```python
from build123d import *

# Parameters (mm, degrees)
SKETCH_1_W          = 10
SKETCH_1_H          = 5
SKETCH_1_W_2        = 30
EXTRUDE_1_DEPTH     = 5
SKETCH_1_3_W        = 10
SKETCH_1_3_H        = 5
SKETCH_1_3_W_2      = 30
EXTRUDE_2_DEPTH     = 85
SKETCH_2_R          = 3
CUT_EXTRUDE_1_DEPTH = 144
FILLET_1_R          = 40
SKETCH_4_W          = 30
SKETCH_4_H          = 5.8
CUT_EXTRUDE_2_DEPTH = 144
SKETCH_5_W          = 60
SKETCH_5_H          = 60
CUT_EXTRUDE_3_DEPTH = 144
SKETCH_6_R          = 5
CUT_EXTRUDE_4_DEPTH = 144


with BuildPart() as part:
    # Sketch 1 → Extrude 1 (new body)
    with BuildSketch(Plane.XY):
        Polygon((0, 42.6), (0, 0), (95, 0), (95, 47.6), (10, 47.6), (10, 42.6), align=None)
        Polygon((10, -42.6), (10, -47.6), (35, -47.6), (75, -47.6), (90, -47.6), (95, -47.6), (95, 0), (0, 0), (0, -42.6), align=None)
        Polygon((35, -47.6), (10, -47.6), (0, -47.6), (0, -52.6), (10, -52.6), (90, -52.6), (95, -52.6), (95, -47.6), (90, -47.6), (75, -47.6), align=None)
        with Locations((5, -45.1)):
            Rectangle(SKETCH_1_W, SKETCH_1_H)
        with Locations((-15, -45.1)):
            Rectangle(SKETCH_1_W_2, SKETCH_1_H)
        Polygon((10, -52.6), (0, -52.6), (-30, -52.6), (-30, -57.6), (10, -57.6), align=None)
        with Locations((-15, 45.1)):
            Rectangle(SKETCH_1_W_2, SKETCH_1_H)
        Polygon((-30, 52.6), (0, 52.6), (10, 52.6), (10, 57.6), (-30, 57.6), align=None)
        Polygon((0, 52.6), (0, 47.6), (10, 47.6), (95, 47.6), (95, 52.6), (10, 52.6), align=None)
        with Locations((5, 45.1)):
            Rectangle(SKETCH_1_W, SKETCH_1_H)
    extrude(amount=-EXTRUDE_1_DEPTH)

    # Sketch 1_3 → Extrude 2 (add)
    with BuildSketch(Plane.XY):
        Polygon((0, 52.6), (0, 47.6), (10, 47.6), (95, 47.6), (95, 52.6), (10, 52.6), align=None)
        Polygon((-30, 52.6), (0, 52.6), (10, 52.6), (10, 57.6), (-30, 57.6), align=None)
        with Locations((5, 45.1)):
            Rectangle(SKETCH_1_3_W, SKETCH_1_3_H)
        with Locations((-15, 45.1)):
            Rectangle(SKETCH_1_3_W_2, SKETCH_1_3_H)
        with Locations((5, -45.1)):
            Rectangle(SKETCH_1_3_W, SKETCH_1_3_H)
        with Locations((-15, -45.1)):
            Rectangle(SKETCH_1_3_W_2, SKETCH_1_3_H)
        Polygon((10, -52.6), (0, -52.6), (-30, -52.6), (-30, -57.6), (10, -57.6), align=None)
        Polygon((35, -47.6), (10, -47.6), (0, -47.6), (0, -52.6), (10, -52.6), (90, -52.6), (95, -52.6), (95, -47.6), (90, -47.6), (75, -47.6), align=None)
    extrude(amount=EXTRUDE_2_DEPTH)

    # Sketch 2 → Cut-Extrude 1 (cut)
    with BuildSketch(Plane.XZ.offset(52.6)):
        with Locations(Location((55, 60, 0), (0, 0, 270))):
            Circle(SKETCH_2_R)
    extrude(amount=-CUT_EXTRUDE_1_DEPTH, mode=Mode.SUBTRACT)

    # Fillet 1
    fillet_1_edges = [part.edges().sort_by_distance(p)[0] for p in [
        (95, -50.1, 85),
        (95, 50.1, 85),
    ]]
    fillet(fillet_1_edges, radius=FILLET_1_R)

    # Sketch 4 → Cut-Extrude 2 (cut)
    with BuildSketch(Plane.XY.offset(85)):
        with Locations((-15, -50.1)):
            Rectangle(SKETCH_4_W, SKETCH_4_H)
        with Locations((-15, 50.1)):
            Rectangle(SKETCH_4_W, SKETCH_4_H)
    extrude(amount=-CUT_EXTRUDE_2_DEPTH, mode=Mode.SUBTRACT)

    # Sketch 5 → Cut-Extrude 3 (cut)
    with BuildSketch(Plane.XY):
        with Locations((45, 0)):
            Rectangle(SKETCH_5_W, SKETCH_5_H)
    extrude(amount=-CUT_EXTRUDE_3_DEPTH, mode=Mode.SUBTRACT)

    # Sketch 6 → Cut-Extrude 4 (cut)
    with BuildSketch(Plane.XZ.offset(57.6)):
        with Locations(Location((-10, 40, 0), (0, 0, 270))):
            Circle(SKETCH_6_R)
        with Locations(Location((-10, 65, 0), (0, 0, 270))):
            Circle(SKETCH_6_R)
        with Locations(Location((-10, 15, 0), (0, 0, 270))):
            Circle(SKETCH_6_R)
    extrude(amount=-CUT_EXTRUDE_4_DEPTH, mode=Mode.SUBTRACT)


solid = part.part
```
Design review of the part built by this model. Coordinates are the model's own, in mm. A direction names the side the tool comes from. Round coordinates to 2 decimals unless told otherwise and drop trailing zeros. Write each loop counter-clockwise with the first axis right and the second up, starting at its lowest first coordinate (ties: lowest second). Pieces come first, ordered by that corner, then holes. Notation, with made-up numbers: (32, -39) -> (76, -39) arc R30 ccw to (76, -17) -> close; hole circle Ø2 at (-3.5, 6). An arc over 180 degrees is marked (long way). Answer in a Markdown table with one row per item.
Q1. Take a section at C-C, the plane x = -19.5. State the section outline as (y, z) points, then the cut area to 3 significant figures.
The answers:
| item | result |
|---|---|
| outline | (-57.6, -5) -> (-53, -5) -> (-53, 85) -> (-57.6, 85) -> close; (-47.2, -5) -> (-42.6, -5) -> (-42.6, 85) -> (-47.2, 85) -> close; (42.6, -5) -> (47.2, -5) -> (47.2, 85) -> (42.6, 85) -> close; (53, -5) -> (57.6, -5) -> (57.6, 85) -> (53, 85) -> close |
| area | 1,660 mm² |
Q2. Clearance check with flat-ended pins moving along their axes: pin 1 Ø5.5 at (y, z) = (-3.5, -1.5) entering from -X; pin 2 Ø4 at (x, z) = (49, -3) entering from +Y; pin 3 Ø3 at (x, z) = (68, 16.5) entering from -Y. State where each tip first meets the part, or that it passes through.
The answers:
| item | result |
|---|---|
| pin 1 | x = 0 |
| pin 2 | y = 52.6 |
| pin 3 | y = -52.6 |
Q3. Take a section at A-A, the plane x = 26. State the section outline as (y, z) points, then the cut area to 3 significant figures.
The answers:
| item | result |
|---|---|
| outline | (-52.6, -5) -> (-30, -5) -> (-30, 0) -> (-47.6, 0) -> (-47.6, 85) -> (-52.6, 85) -> close; (30, -5) -> (52.6, -5) -> (52.6, 85) -> (47.6, 85) -> (47.6, 0) -> (30, 0) -> close |
| area | 1,080 mm² |
Q4. Take a section at D-D, the plane z = 78. State the section outline as (x, y) points.
The answers:
| item | result |
|---|---|
| outline | (-30, -57.6) -> (10, -57.6) -> (10, -52.6) -> (77.61, -52.6) -> (77.61, -47.6) -> (10, -47.6) -> (10, -42.6) -> (-30, -42.6) -> (-30, -47.2) -> (0, -47.2) -> (0, -53) -> (-30, -53) -> close; (-30, 42.6) -> (10, 42.6) -> (10, 47.6) -> (77.61, 47.6) -> (77.61, 52.6) -> (10, 52.6) -> (10, 57.6) -> (-30, 57.6) -> (-30, 53) -> (0, 53) -> (0, 47.2) -> (-30, 47.2) -> close |
Q5. Take a section at B-B, the plane y = 16. State the section outline as (x, z) points.
The answers:
| item | result |
|---|---|
| outline | (0, -5) -> (15, -5) -> (15, 0) -> (0, 0) -> close; (75, -5) -> (95, -5) -> (95, 0) -> (75, 0) -> close |
Q6. Draft analysis for pull direction Z (two halves, no side actions). For faces 1 (the face through (10, 45, 42)), 2 (the face through (82.972, 50.135, 73.594)), 3 (the face through (-7, 45, 19)), state which applies: +Z half, -Z half, draft (parallel to the pull), parting line (faces both ways), or undercut.
The answers:
| item | result |
|---|---|
| face 1 | draft |
| face 2 | +Z half |
| face 3 | undercut |
Q7. To check wall thickness, follow L1, parallel to Y at x = -20, z = 79.5; L2, parallel to Y at x = 14, z = 34.5; L3, parallel to X at y = 55.45, z = 65. State the ranges of each line that lie inside material, in increasing order. Write a range as [from, to].
The answers:
| item | result |
|---|---|
| L1 | [-57.6, -53], [-47.2, -42.6], [42.6, 47.2], [53, 57.6] |
| L2 | [-52.6, -47.6], [47.6, 52.6] |
| L3 | [-30, -15], [-5, 10] |
Q8. For faces 4 (the face through (-15.2, 47.2, 40.6)), 5 (the face through (53, -47.6, 42)), 6 (the face through (52, -52.6, 41)), list the 3-axis set-ups (+Z, -Z, +X, -X, +Y, -Y) from which the entire face can be reached by the end or side of a thin tool; tool diameter is ignored.
The answers:
| item | result |
|---|---|
| face 4 | +Z, -Z, -X |
| face 5 | +Z, +X |
| face 6 | +Z, -Z, +X, -Y |
